CAD build for the part. Positions are in the model's coordinates, mm. A direction names the side the tool comes from. Round coordinates to 2 decimals unless told otherwise and drop trailing zeros. Order: outer loops, then holes, each group sorted by start corner. A loop starts at its lowest first (then second) coordinate and runs counter-clockwise, first axis right, second up. Notation, with made-up numbers: M -15,46.25 L -6,46.25 A9 cw -6,56.25 Z; hole C 52,-6 d9. An arc over 180 degrees is marked long. Answer as a JSON object with one key per item and string values.
```python
from build123d import *

# Parameters (mm, degrees)
F0_R     = 5
F0_R_2   = 1.9
F1_DEPTH = 15
F2_DEPTH = 10
F3_R     = 3.962687
F4_DEPTH = 5
F3_R_2   = 1.9
F5_DEPTH = 9


with BuildPart() as f1:
    # F0 (on Top) → F1 (new body)
    with BuildSketch(Plane.XY):
        Circle(F0_R)
        Circle(F0_R_2, mode=Mode.SUBTRACT)
    extrude(amount=F1_DEPTH)

    # F0 (on Top) → F2 (join)
    with BuildSketch(Plane.XY):
        with BuildLine():
            ThreePointArc((6.487681, -0.4), (6.496919, -0.200095), (6.5, 0))
            ThreePointArc((6.5, 0), (6.496919, 0.200095), (6.487681, 0.4))
            ThreePointArc((6.487681, 0.4), (6.419974, 1.016824), (6.293758, 1.624381))
            ThreePointArc((6.293758, 1.624381), (6.181867, 2.00861), (6.046544, 2.385226))
            ThreePointArc((6.046544, 2.385226), (5.791542, 2.950938), (5.483758, 3.489756))
            ThreePointArc((5.483758, 3.489756), (5.25861, 3.820604), (5.01353, 4.13697))
            ThreePointArc((5.01353, 4.13697), (4.596194, 4.596194), (4.13697, 5.01353))
            ThreePointArc((4.13697, 5.01353), (3.820604, 5.25861), (3.489756, 5.483758))
            ThreePointArc((3.489756, 5.483758), (2.950938, 5.791542), (2.385226, 6.046544))
            ThreePointArc((2.385226, 6.046544), (2.00861, 6.181867), (1.624381, 6.293758))
            ThreePointArc((1.624381, 6.293758), (1.016824, 6.419974), (0.4, 6.487681))
            ThreePointArc((0.4, 6.487681), (0, 6.5), (-0.4, 6.487681))
            ThreePointArc((-0.4, 6.487681), (-1.016824, 6.419974), (-1.624381, 6.293758))
            ThreePointArc((-1.624381, 6.293758), (-2.00861, 6.181867), (-2.385226, 6.046544))
            ThreePointArc((-2.385226, 6.046544), (-2.950938, 5.791542), (-3.489756, 5.483758))
            ThreePointArc((-3.489756, 5.483758), (-3.820604, 5.25861), (-4.13697, 5.01353))
            ThreePointArc((-4.13697, 5.01353), (-4.596194, 4.596194), (-5.01353, 4.13697))
            ThreePointArc((-5.01353, 4.13697), (-5.25861, 3.820604), (-5.483758, 3.489756))
            ThreePointArc((-5.483758, 3.489756), (-5.791542, 2.950938), (-6.046544, 2.385226))
            ThreePointArc((-6.046544, 2.385226), (-6.181867, 2.00861), (-6.293758, 1.624381))
            ThreePointArc((-6.293758, 1.624381), (-6.419974, 1.016824), (-6.487681, 0.4))
            ThreePointArc((-6.487681, 0.4), (-6.5, 0), (-6.487681, -0.4))
            ThreePointArc((-6.487681, -0.4), (-6.419974, -1.016824), (-6.293758, -1.624381))
            ThreePointArc((-6.293758, -1.624381), (-6.181867, -2.00861), (-6.046544, -2.385226))
            ThreePointArc((-6.046544, -2.385226), (-5.791542, -2.950938), (-5.483758, -3.489756))
            ThreePointArc((-5.483758, -3.489756), (-5.25861, -3.820604), (-5.01353, -4.13697))
            ThreePointArc((-5.01353, -4.13697), (-4.596194, -4.596194), (-4.13697, -5.01353))
            ThreePointArc((-4.13697, -5.01353), (-3.820604, -5.25861), (-3.489756, -5.483758))
            ThreePointArc((-3.489756, -5.483758), (-2.950938, -5.791542), (-2.385226, -6.046544))
            ThreePointArc((-2.385226, -6.046544), (-2.00861, -6.181867), (-1.624381, -6.293758))
            ThreePointArc((-1.624381, -6.293758), (-1.016824, -6.419974), (-0.4, -6.487681))
            ThreePointArc((-0.4, -6.487681), (0, -6.5), (0.4, -6.487681))
            ThreePointArc((0.4, -6.487681), (1.016824, -6.419974), (1.624381, -6.293758))
            ThreePointArc((1.624381, -6.293758), (2.00861, -6.181867), (2.385226, -6.046544))
            ThreePointArc((2.385226, -6.046544), (2.950938, -5.791542), (3.489756, -5.483758))
            ThreePointArc((3.489756, -5.483758), (3.820604, -5.25861), (4.13697, -5.01353))
            ThreePointArc((4.13697, -5.01353), (4.596194, -4.596194), (5.01353, -4.13697))
            ThreePointArc((5.01353, -4.13697), (5.25861, -3.820604), (5.483758, -3.489756))
            ThreePointArc((5.483758, -3.489756), (5.791542, -2.950938), (6.046544, -2.385226))
            ThreePointArc((6.046544, -2.385226), (6.181867, -2.00861), (6.293758, -1.624381))
            ThreePointArc((6.293758, -1.624381), (6.419974, -1.016824), (6.487681, -0.4))
        make_face()
        Circle(F0_R, mode=Mode.SUBTRACT)
        with BuildLine():
            ThreePointArc((-5.483758, 3.489756), (-5.25861, 3.820604), (-5.01353, 4.13697))
            Line((-5.01353, 4.13697), (-5.822547, 4.724755))
            Line((-5.822547, 4.724755), (-6.292775, 4.077541))
            Line((-6.292775, 4.077541), (-5.483758, 3.489756))
        make_face()
        with BuildLine():
            ThreePointArc((-4.13697, 5.01353), (-3.820604, 5.25861), (-3.489756, 5.483758))
            Line((-3.489756, 5.483758), (-4.077541, 6.292775))
            Line((-4.077541, 6.292775), (-4.724755, 5.822547))
            Line((-4.724755, 5.822547), (-4.13697, 5.01353))
        make_face()
        with BuildLine():
            ThreePointArc((-6.487681, -0.4), (-6.5, 0), (-6.487681, 0.4))
            Line((-6.487681, 0.4), (-7.487681, 0.4))
            Line((-7.487681, 0.4), (-7.487681, -0.4))
            Line((-7.487681, -0.4), (-6.487681, -0.4))
        make_face()
        with BuildLine():
            Line((-6.997601, -2.694243), (-6.046544, -2.385226))
            ThreePointArc((-6.046544, -2.385226), (-6.181867, -2.00861), (-6.293758, -1.624381))
            Line((-6.293758, -1.624381), (-7.244814, -1.933398))
            Line((-7.244814, -1.933398), (-6.997601, -2.694243))
        make_face()
        with BuildLine():
            ThreePointArc((-6.293758, 1.624381), (-6.181867, 2.00861), (-6.046544, 2.385226))
            Line((-6.046544, 2.385226), (-6.997601, 2.694243))
            Line((-6.997601, 2.694243), (-7.244814, 1.933398))
            Line((-7.244814, 1.933398), (-6.293758, 1.624381))
        make_face()
        with BuildLine():
            Line((-5.822547, -4.724755), (-5.01353, -4.13697))
            ThreePointArc((-5.01353, -4.13697), (-5.25861, -3.820604), (-5.483758, -3.489756))
            Line((-5.483758, -3.489756), (-6.292775, -4.077541))
            Line((-6.292775, -4.077541), (-5.822547, -4.724755))
        make_face()
        with BuildLine():
            Line((-4.077541, -6.292775), (-3.489756, -5.483758))
            ThreePointArc((-3.489756, -5.483758), (-3.820604, -5.25861), (-4.13697, -5.01353))
            Line((-4.13697, -5.01353), (-4.724755, -5.822547))
            Line((-4.724755, -5.822547), (-4.077541, -6.292775))
        make_face()
        with BuildLine():
            Line((-1.933398, -7.244814), (-1.624381, -6.293758))
            ThreePointArc((-1.624381, -6.293758), (-2.00861, -6.181867), (-2.385226, -6.046544))
            Line((-2.385226, -6.046544), (-2.694243, -6.997601))
            Line((-2.694243, -6.997601), (-1.933398, -7.244814))
        make_face()
        with BuildLine():
            Line((0.4, -7.487681), (0.4, -6.487681))
            ThreePointArc((0.4, -6.487681), (0, -6.5), (-0.4, -6.487681))
            Line((-0.4, -6.487681), (-0.4, -7.487681))
            Line((-0.4, -7.487681), (0.4, -7.487681))
        make_face()
        with BuildLine():
            Line((2.694243, -6.997601), (2.385226, -6.046544))
            ThreePointArc((2.385226, -6.046544), (2.00861, -6.181867), (1.624381, -6.293758))
            Line((1.624381, -6.293758), (1.933398, -7.244814))
            Line((1.933398, -7.244814), (2.694243, -6.997601))
        make_face()
        with BuildLine():
            Line((4.724755, -5.822547), (4.13697, -5.01353))
            ThreePointArc((4.13697, -5.01353), (3.820604, -5.25861), (3.489756, -5.483758))
            Line((3.489756, -5.483758), (4.077541, -6.292775))
            Line((4.077541, -6.292775), (4.724755, -5.822547))
        make_face()
        with BuildLine():
            Line((7.244814, -1.933398), (6.293758, -1.624381))
            ThreePointArc((6.293758, -1.624381), (6.181867, -2.00861), (6.046544, -2.385226))
            Line((6.046544, -2.385226), (6.997601, -2.694243))
            Line((6.997601, -2.694243), (7.244814, -1.933398))
        make_face()
        with BuildLine():
            ThreePointArc((6.487681, 0.4), (6.496919, 0.200095), (6.5, 0))
            ThreePointArc((6.5, 0), (6.496919, -0.200095), (6.487681, -0.4))
            Line((6.487681, -0.4), (7.487681, -0.4))
            Line((7.487681, -0.4), (7.487681, 0.4))
            Line((7.487681, 0.4), (6.487681, 0.4))
        make_face()
        with BuildLine():
            ThreePointArc((6.046544, 2.385226), (6.181867, 2.00861), (6.293758, 1.624381))
            Line((6.293758, 1.624381), (7.244814, 1.933398))
            Line((7.244814, 1.933398), (6.997601, 2.694243))
            Line((6.997601, 2.694243), (6.046544, 2.385226))
        make_face()
        with BuildLine():
            ThreePointArc((3.489756, 5.483758), (3.820604, 5.25861), (4.13697, 5.01353))
            Line((4.13697, 5.01353), (4.724755, 5.822547))
            Line((4.724755, 5.822547), (4.077541, 6.292775))
            Line((4.077541, 6.292775), (3.489756, 5.483758))
        make_face()
        with BuildLine():
            Line((6.292775, -4.077541), (5.483758, -3.489756))
            ThreePointArc((5.483758, -3.489756), (5.25861, -3.820604), (5.01353, -4.13697))
            Line((5.01353, -4.13697), (5.822547, -4.724755))
            Line((5.822547, -4.724755), (6.292775, -4.077541))
        make_face()
        with BuildLine():
            ThreePointArc((5.01353, 4.13697), (5.25861, 3.820604), (5.483758, 3.489756))
            Line((5.483758, 3.489756), (6.292775, 4.077541))
            Line((6.292775, 4.077541), (5.822547, 4.724755))
            Line((5.822547, 4.724755), (5.01353, 4.13697))
        make_face()
        with BuildLine():
            ThreePointArc((1.624381, 6.293758), (2.00861, 6.181867), (2.385226, 6.046544))
            Line((2.385226, 6.046544), (2.694243, 6.997601))
            Line((2.694243, 6.997601), (1.933398, 7.244814))
            Line((1.933398, 7.244814), (1.624381, 6.293758))
        make_face()
        with BuildLine():
            ThreePointArc((-2.385226, 6.046544), (-2.00861, 6.181867), (-1.624381, 6.293758))
            Line((-1.624381, 6.293758), (-1.933398, 7.244814))
            Line((-1.933398, 7.244814), (-2.694243, 6.997601))
            Line((-2.694243, 6.997601), (-2.385226, 6.046544))
        make_face()
        with BuildLine():
            ThreePointArc((-0.4, 6.487681), (0, 6.5), (0.4, 6.487681))
            Line((0.4, 6.487681), (0.4, 7.487681))
            Line((0.4, 7.487681), (-0.4, 7.487681))
            Line((-0.4, 7.487681), (-0.4, 6.487681))
        make_face()
    extrude(amount=F2_DEPTH)

    # F3 (on face) → F4 (cut)
    with BuildSketch(Plane.XY):
        Circle(F3_R)
        Polygon((-2.7, 1.558846), (0, 3.117691), (2.7, 1.558846), (2.7, -1.558846), (0, -3.117691), (-2.7, -1.558846), align=None, mode=Mode.SUBTRACT)
    extrude(amount=F4_DEPTH, mode=Mode.SUBTRACT)

    # F3 (on face) → F5 (cut)
    with BuildSketch(Plane.XY):
        Polygon((2.7, 1.558846), (0, 3.117691), (-2.7, 1.558846), (-2.7, -1.558846), (0, -3.117691), (2.7, -1.558846), align=None)
        Circle(F3_R_2, mode=Mode.SUBTRACT)
    extrude(amount=F5_DEPTH, mode=Mode.SUBTRACT)


solid = f1.part
```
Item 1: Saw through at C-C on x = 1.25. List the corners of the cut face in (y, z), and give its area (3 significant figures).
Worked answers:
{"outline": "M -6.38,0 L -3.76,0 L -3.76,5 L -2.4,5 L -2.4,9 L -1.43,9 L -1.43,15 L -4.84,15 L -4.84,10 L -6.38,10 Z; M 1.43,9 L 2.4,9 L 2.4,5 L 3.76,5 L 3.76,0 L 6.38,0 L 6.38,10 L 4.84,10 L 4.84,15 L 1.43,15 Z", "area": "102 mm2"}
Item 2: Drop flat-ended pins along their axis: pin 1 Ø6 at (x, y) = (1, 0) entering from -Z; pin 2 Ø1.1 at (x, z) = (7, 4) entering from -Y; pin 3 Ø0.8 at (x, z) = (-7, 2.5) entering from +Y; pin 4 Ø7 at (x, y) = (0, 0) entering from -Z. Give the stop position or say it passes through.
Worked answers:
{"pin 1": "stops at z = 0", "pin 2": "stops at y = -2.69", "pin 3": "stops at y = 2.69", "pin 4": "stops at z = 5"}
Item 3: Saw through at A-A on y = 0. List the corners of the cut face in (x, z), and give its area (3 significant figures).
Worked answers:
{"outline": "M -7.49,0 L -3.96,0 L -3.96,5 L -2.7,5 L -2.7,9 L -1.9,9 L -1.9,15 L -5,15 L -5,10 L -7.49,10 Z; M 1.9,9 L 2.7,9 L 2.7,5 L 3.96,5 L 3.96,0 L 7.49,0 L 7.49,10 L 5,10 L 5,15 L 1.9,15 Z", "area": "116 mm2"}
Item 4: Two-plate mould, pull along Y, no slides. Class faces 6 (the flat face through (-5.42, -4.43, 4.93)), 7 (the flat face through (-1.369, -2.327, 6.972)), 8 (the flat face through (-3.4, 3.9, 10)), 9 (the cylindrical face through (-1.01, 6.42, 4.93)): released by +Y, released by -Y, zero draft, split by the parting line, or undercut.
Worked answers:
{"face 6": "released by -Y", "face 7": "undercut", "face 8": "zero draft", "face 9": "released by +Y"}
Item 5: Saw through at D-D on x = 3. List the corners of the cut face in (y, z), and give its area (3 significant figures).
Worked answers:
{"outline": "M -5.77,0 L -2.59,0 L -2.59,5 L 2.59,5 L 2.59,0 L 5.77,0 L 5.77,10 L 4,10 L 4,15 L -4,15 L -4,10 L -5.77,10 Z", "area": "129 mm2"}
Item 6: Wall check: line 1 along Y through (x, z) = (0, 1.8); line 2 along Y through (x, z) = (0, 10.8); line 3 along Z through (x, y) = (-0.5, 5.5). Give the ranges that are in metal, low to high. Write a range as [from, to].
Worked answers:
{"line 1": "y = [-7.49, -3.96], [3.96, 7.49]", "line 2": "y = [-5, -1.9], [1.9, 5]", "line 3": "z = [0, 10]"}
Item 7: Saw through at B-B on y = 6.75. List the corners of the cut face in (x, z).
Worked answers:
{"outline": "M -2.61,0 L -1.77,0 L -1.77,10 L -2.61,10 Z; M -0.4,0 L 0.4,0 L 0.4,10 L -0.4,10 Z; M 1.77,0 L 2.61,0 L 2.61,10 L 1.77,10 Z"}
Item 8: 3-axis set-ups, long thin cutter, end or side, ignore diameter. For faces 1 (the flat face through (7, -0.4, 5)), 2 (the flat face through (-5.88, -3.78, 4.93)), 3 (the flat face through (6.529, 2.542, 4.93)), 4 (the cylindrical face through (1.025, 6.419, 4.93)), 5 (the flat face through (1.369, 2.327, 6.972)): which of +Z, -Z, +X, -X, +Y, -Y reach the whole face in a straight line?
Worked answers:
{"face 1": "+Z, -Z, +X", "face 2": "+Z, -Z, -X", "face 3": "+Z, -Z", "face 4": "+Z, -Z, +Y", "face 5": "-Z"}
